Design review of the part built by this model. Coordinates are the model's own, in mm. A direction names the side the tool comes from. Give positions to 0.01 mm unless a question says otherwise; leave off trailing zeros. Order: outer loops, then holes, each group sorted by start corner. A loop starts at its lowest first (then second) coordinate and runs counter-clockwise, first axis right, second up. Notation, with made-up numbers: (-8, 17) -> (3, 17) arc R12 ccw to (3, 38) -> close; hole circle Ø7 at (35, 32). An arc over 180 degrees is marked (long way). Return JSON: item names as keys, results as strings.
```python
from build123d import *

# Parameters (mm, degrees)
F0_W     = 20
F0_H     = 20
F0_R     = 2.15
F2_DEPTH = 25
F3_DEPTH = 25.001
F4_R     = 1.5
F5_R     = 0.5


with BuildPart() as f2:
    # F0 (on Top) → F2 (new body)
    with BuildSketch(Plane.XY):
        Rectangle(F0_W, F0_H)
        Circle(F0_R, mode=Mode.SUBTRACT)
    extrude(amount=F2_DEPTH)

    # F1 (on face) → F3 (cut, through all)
    with BuildSketch(Plane.XY):
        Polygon((-8.5, 2.63), (-10, 2.63), (-10, -2.63), (-8.5, -2.63), (-8.5, -6), (-7.06066, -6), (-3.65, -2.58934), (-3.65, 2.58934), (-7.06066, 6), (-8.5, 6), align=None)
        Polygon((-2.63, -8.5), (-2.63, -10), (2.63, -10), (2.63, -8.5), (6, -8.5), (6, -7.06066), (2.58934, -3.65), (-2.58934, -3.65), (-6, -7.06066), (-6, -8.5), align=None)
        Polygon((10, -2.63), (10, 2.63), (8.5, 2.63), (8.5, 6), (7.06066, 6), (3.65, 2.58934), (3.65, -2.58934), (7.06066, -6), (8.5, -6), (8.5, -2.63), align=None)
        Polygon((2.63, 10), (-2.63, 10), (-2.63, 8.5), (-6, 8.5), (-6, 7.06066), (-2.58934, 3.65), (2.58934, 3.65), (6, 7.06066), (6, 8.5), (2.63, 8.5), align=None)
    extrude(amount=F3_DEPTH, mode=Mode.SUBTRACT)

    # F4
    f4_edges = [f2.edges().sort_by_distance(p)[0] for p in [
        (10, -10, 12.5),
        (-10, -10, 12.5),
        (10, 10, 12.5),
        (-10, 10, 12.5),
    ]]
    fillet(f4_edges, radius=F4_R)

    # F5
    f5_edges = [f2.edges().sort_by_distance(p)[0] for p in [
        (-2.63, -10, 12.5),
        (-10, 2.63, 12.5),
        (-2.63, 10, 12.5),
        (2.63, -10, 12.5),
        (10, 2.63, 12.5),
        (10, -2.63, 12.5),
        (-10, -2.63, 12.5),
        (2.63, 10, 12.5),
        (-6, -8.5, 12.5),
        (-2.63, -8.5, 12.5),
        (2.63, -8.5, 12.5),
        (-8.5, 2.63, 12.5),
        (-8.5, -2.63, 12.5),
        (8.5, -2.63, 12.5),
        (8.5, 2.63, 12.5),
        (2.63, 8.5, 12.5),
        (6, 8.5, 12.5),
        (8.5, 6, 12.5),
        (7.06066, 6, 12.5),
        (6, 7.06066, 12.5),
        (-2.58934, -3.65, 12.5),
        (2.58934, -3.65, 12.5),
        (3.65, 2.58934, 12.5),
        (3.65, -2.58934, 12.5),
        (-3.65, -2.58934, 12.5),
        (-3.65, 2.58934, 12.5),
        (2.58934, 3.65, 12.5),
        (-2.58934, 3.65, 12.5),
        (-6, 8.5, 12.5),
        (-6, 7.06066, 12.5),
        (-2.63, 8.5, 12.5),
        (8.5, -6, 12.5),
        (7.06066, -6, 12.5),
        (-8.5, -6, 12.5),
        (-7.06066, -6, 12.5),
        (-6, -7.06066, 12.5),
        (6, -7.06066, 12.5),
        (6, -8.5, 12.5),
        (-8.5, 6, 12.5),
        (-7.06066, 6, 12.5),
    ]]
    fillet(f5_edges, radius=F5_R)


solid = f2.part
```
Item 1: Add section A-A (x = 0). Give the boundary of the cut face in (y, z), plus the area to 3 significant figures.
Result set:
{"outline": "(-3.65, 0) -> (-2.15, 0) -> (-2.15, 25) -> (-3.65, 25) -> close; (2.15, 0) -> (3.65, 0) -> (3.65, 25) -> (2.15, 25) -> close", "area": "75.0 mm^2"}
Item 2: Mouldability with a two-part tool opening along Y and no side actions: class faces 1 (the face through (-9.57, -9.55, 12.68)), 2 (the face through (-6, 10, 12)), 3 (the face through (-8.5, 4, 12)) as released by +Y, released by -Y, zero draft, split by the parting line, or undercut.
Result set:
{"face 1": "released by -Y", "face 2": "released by +Y", "face 3": "undercut"}
Item 3: Wall thickness on L1, parallel to Y at x = 0, z = 6.75; L2, parallel to Y at x = -4.25, z = 10.25; L3, parallel to X at y = -5.5, z = 7.75: over which ranges is each line inside the solid? List them lowest first. Write a range as [from, to].
Result set:
{"L1": "y = [-3.65, -2.15], [2.15, 3.65]", "L2": "y = [-10, -8.5], [-5.31, -3.19], [3.19, 5.31], [8.5, 10]", "L3": "x = [-10, -8.5], [-6.56, -4.44], [4.44, 6.56], [8.5, 10]"}
Item 4: For pin 1 (1.4 mm diameter, centred on x = -0.5, z = 14, fed in from +Y); pin 2 (1.5 mm diameter, centred on y = 0.5, z = 16, fed in from +X); pin 3 (2.5 mm diameter, centred on x = -1, z = 17.5, fed in from -Y); pin 4 (4 mm diameter, centred on y = 2.5, z = 8, fed in from -X), all flat-tipped, find the tip position at first contact; note any pin that passes through.
Result set:
{"pin 1": "stops at y = 3.65", "pin 2": "stops at x = 3.65", "pin 3": "stops at y = -3.65", "pin 4": "stops at x = -10"}
Item 5: Machinability: for faces 4 (the face through (3.65, 0, 12)), 5 (the face through (-5.38, -4.32, 12.32)), 6 (the face through (-0.1, 2.4, 0)), which of the approach directions +Z, -Z, +X, -X, +Y, -Y give a long, thin tool a straight path to every point of the face, cutting with its end or side? Answer none if there is none.
Result set:
{"face 4": "+Z, -Z, +X", "face 5": "+Z, -Z", "face 6": "-Z, +X, -X, +Y, -Y"}
